from build123d import *

# Parameters (mm, degrees)
BOSS_EXTRU_1_DEPTH = 100


with BuildPart() as part:
    # Esquisse1 → Boss.-Extru.1 (new body)
    with BuildSketch(Plane.XY):
        with BuildLine():
            Line((-26, 0), (-24, 0))
            ThreePointArc((-24, 0), (0, 24), (24, 0))
            Line((24, 0), (26, 0))
            ThreePointArc((26, 0), (18.384776311, 18.384776311), (0, 26))
            ThreePointArc((0, 26), (-18.384776311, 18.384776311), (-26, 0))
        make_face()
    extrude(amount=BOSS_EXTRU_1_DEPTH)


solid = part.part
Build history of the part. All positions in model axes, mm. Round coordinates to 2 decimals unless told otherwise and drop trailing zeros. Loops run counter-clockwise (first coordinate to the right, second up) from the corner with the lowest first, then second, coordinate; pieces in that order, holes last. Notation, with made-up numbers: (80.25, 14) -> (121.25, 14) arc R29 ccw to (121.25, 46) -> close; hole circle Ø6 at (44, 55). An arc over 180 degrees is marked (long way). Answer in a Markdown table with one row per item.
Item 1: Saw through at C-C (y = 10). Write the cut outline in (x, z).
Answers below:
| item | result |
|---|---|
| outline | (-24, 0) -> (-21.82, 0) -> (-21.82, 100) -> (-24, 100) -> close; (21.82, 0) -> (24, 0) -> (24, 100) -> (21.82, 100) -> close |
Item 2: Drill centre lines: L1, parallel to Y at x = 1, z = 77; L2, parallel to X at y = 15.5, z = 85; L3, parallel to X at y = 16.5, z = 28.5. Where is each one in solid material? Low to high. Write a range as [from, to].
Answers below:
| item | result |
|---|---|
| L1 | y = [23.98, 25.98] |
| L2 | x = [-20.87, -18.32], [18.32, 20.87] |
| L3 | x = [-20.09, -17.43], [17.43, 20.09] |
Item 3: Saw through at D-D (x = 9.5). Write the cut outline in (y, z).
Answers below:
| item | result |
|---|---|
| outline | (22.04, 0) -> (24.2, 0) -> (24.2, 100) -> (22.04, 100) -> close |
Item 4: Mould opens along X. For faces 1 (the cylindrical face through (-0.528, 23.994, 49.3)), 2 (the flat face through (0, 25, 100)) say: +X half, -X half, draft (parallel to the pull), parting line (faces both ways), or undercut.
Answers below:
| item | result |
|---|---|
| face 1 | undercut |
| face 2 | draft |
Item 5: Saw through at A-A (y = 22). Write the cut outline in (x, z).
Answers below:
| item | result |
|---|---|
| outline | (-13.86, 0) -> (-9.59, 0) -> (-9.59, 100) -> (-13.86, 100) -> close; (9.59, 0) -> (13.86, 0) -> (13.86, 100) -> (9.59, 100) -> close |
Item 6: Pin check, flat tips, straight feed: pin 1 (4 mm diameter, centred on y = 15, z = 44, fed in from +X); pin 2 (3 mm diameter, centred on x = 14, z = 66, fed in from +Y); pin 3 (4 mm diameter, centred on x = -14.5, z = 78.5, fed in from -Y). Stop position of each tip, or through.
Answers below:
| item | result |
|---|---|
| pin 1 | stops at x = 22.52 |
| pin 2 | stops at y = 22.8 |
| pin 3 | stops at y = 17.43 |
Item 7: Saw through at B-B (z = 65.5). Write the cut outline in (x, y), and give its area (3 significant figures).
Answers below:
| item | result |
|---|---|
| outline | (-26, 0) -> (-24, 0) arc R24 cw to (24, 0) -> (26, 0) arc R26 ccw to start |
| area | 157 mm² |
